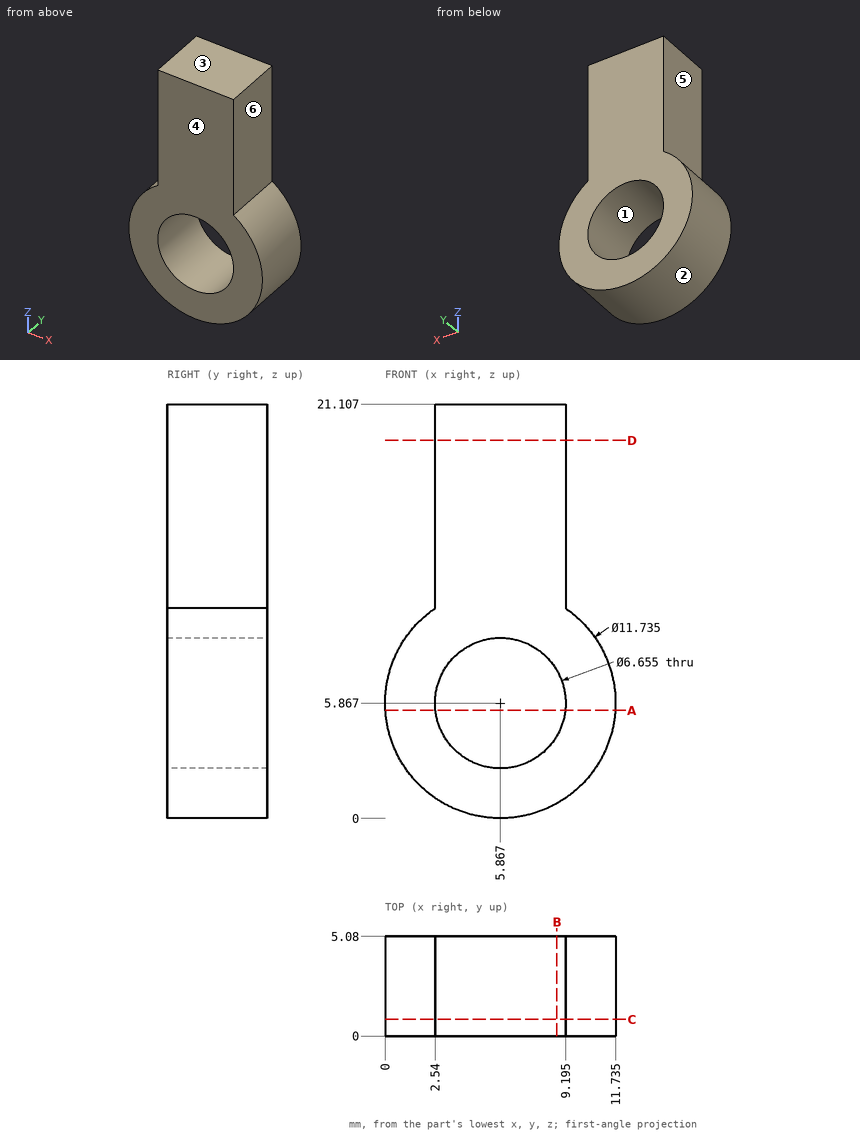
Could you check a few things on this drawing? It's one solid part, dimensions in mm from its lowest x, y, z. A direction names the side the tool comes from. Coordinates: 2 decimals unless noted, no trailing zeros. Order: outer loops, then holes, each group sorted by start corner. A loop starts at its lowest first (then second) coordinate and runs counter-clockwise, first axis right, second up. Notation, with made-up numbers: (69.25, 16.25) -> (89.25, 16.25) arc R22 cw to (89.25, 45.25) -> close; hole circle Ø8 at (-6.75, 41.25). An arc over 180 degrees is marked (long way). Answer in a Markdown table with one row per item.
(1) I want a section at A-A on z = 5.5. List the corners of the cut face in (x, y) for me (1 decimal).
Answer key:
| item | result |
|---|---|
| outline | (0, 0) -> (2.6, 0) -> (2.6, 5.1) -> (0, 5.1) -> close; (9.2, 0) -> (11.7, 0) -> (11.7, 5.1) -> (9.2, 5.1) -> close |
(2) I want a section at B-B on x = 8.75. List the corners of the cut face in (y, z) for me (1 decimal).
Answer key:
| item | result |
|---|---|
| outline | (0, 0.8) -> (5.1, 0.8) -> (5.1, 4.2) -> (0, 4.2) -> close; (0, 7.5) -> (5.1, 7.5) -> (5.1, 21.1) -> (0, 21.1) -> close |
(3) I want a section at D-D on z = 19.25. List the corners of the cut face in (x, y) for me (1 decimal), then the cut area to 3 significant figures.
Answer key:
| item | result |
|---|---|
| outline | (2.5, 0) -> (9.2, 0) -> (9.2, 5.1) -> (2.5, 5.1) -> close |
| area | 33.8 mm^2 |
(4) I want a section at C-C on y = 0.85. List the corners of the cut face in (x, z) for me (1 decimal), then the cut area to 3 significant figures.
Answer key:
| item | result |
|---|---|
| outline | (2.5, 10.7) arc R5.9 ccw (long way) to (9.2, 10.7) -> (9.2, 21.1) -> (2.5, 21.1) -> close; hole circle Ø6.7 at (5.9, 5.9) |
| area | 138 mm^2 |
(5) Please list where these lines run through material, in increasing order: probe 1 along X at (y, z) = (4.35, 6); probe 2 along Z at (x, y) = (5.75, 1.5); probe 3 along Z at (x, y) = (8.5, 1.45) (1 decimal).
Answer key:
| item | result |
|---|---|
| probe 1 | 0 to 2.54, 9.19 to 11.73 |
| probe 2 | 0 to 2.54, 9.19 to 21.11 |
| probe 3 | 0.6 to 3.8, 7.9 to 21.1 |
(6) On a 3-axis mill with a long thin cutter (end or side, diameter ignored), from which of +Z, -Z, +X, -X, +Y, -Y can I reach the whole of each face in a straight line? I mean the marked faces 4, 5 and 6. Say none if no direction works.
Answer key:
| item | result |
|---|---|
| face 4 | +Z, -Z, +X, -X, -Y |
| face 5 | +Z, -X, +Y, -Y |
| face 6 | +Z, +X, +Y, -Y |
(7) Thinking about a two-plate mould opening in X: for the marked faces 1, 2 and 3, which applies, +X half, -X half, draft (parallel to the pull), parting line (faces both ways), or undercut?
Answer key:
| item | result |
|---|---|
| face 1 | undercut |
| face 2 | parting line |
| face 3 | draft |
